For this review, take the finished solid that the model builds, in its own axes (mm). A direction names the side the tool comes from. Round coordinates to 2 decimals unless told otherwise and drop trailing zeros. Loops run counter-clockwise (first coordinate to the right, second up) from the corner with the lowest first, then second, coordinate; pieces in that order, holes last.
1) Mouldability with a two-part tool opening along X and no side actions: class faces 1 (the cylindrical face through (21.107, 38.24, 23.706)), 2 (the flat face through (24.237, 75, 21)), 3 (the flat face through (-20.213, 75, 20)) as pulls with the +X half, pulls with the -X half, needs draft (parallel to the pull), parting line crosses it, or undercut.
2) Take a section at A-A (x = -16.5). State the section outline as (y, z) points, then the cut area to 3 significant figures.
3) Take a section at B-B (y = 63.5). State the section outline as (x, z) points.
4) Take a section at D-D (z = 21.75). Give the number of separate pieces and of enclosed holes in the cut face, then the cut area to 3 significant figures.
5) Wall thickness on L1, parallel to Z at x = -18.5, y = 55.5; L2, parallel to X at y = 126, z = 17.75; L3, parallel to Z at x = -24, y = 12.5: over which ranges is each line inside the solid? List them lowest first.
6) Take a section at C-C (y = 24). State the section outline as (x, z) points, then the cut area to 3 significant figures.
7) Tool access review of faces 4 (the cylindrical face through (21.11, 85.8, 21.22)), 5 (the flat face through (-1, 75, 26.884)): name each direction out of +Z, -Z, +X, -X, +Y, -Y from which nothing blocks a thin tool from reaching the whole face with its end or side.
Autodesk Inventor part; units mm, degrees
ref_plane "YZ Plane" through (0, 0, 0) normal (1, 0, 0) x (0, 1, 0)
ref_plane "XZ Plane" through (0, 0, 0) normal (0, 1, 0) x (-1, 0, 0)
ref_plane "XY Plane" through (0, 0, 0) normal (0, 0, 1) x (1, 0, 0)
sketch "Sketch1" plane through (0, 0, 0) normal (0, 1, 0) x (-1, 0, 0)
  line L0 (-24.2371, 7.8342) -> (26.5629, 7.8342)
  line L1 (26.5629, 7.8342) -> (26.5629, 33.2342)
  line L2 (26.5629, 33.2342) -> (-24.2371, 33.2342)
  line L3 (-24.2371, 33.2342) -> (-24.2371, 7.8342)
  line L4 (-17.8871, 14.1842) -> (20.2129, 14.1842)
  line L5 (20.2129, 14.1842) -> (20.2129, 26.8842)
  line L6 (20.2129, 26.8842) -> (-17.8871, 26.8842)
  line L7 (-17.8871, 26.8842) -> (-17.8871, 14.1842)
  point P0 (0, 0)
  dimension "d0" = 50.8
  dimension "d1" = 25.4
  dimension "d2" = 6.35
extrude "Extrusion1" add sketch "Sketch1" along normal blind 152.4
sketch "Sketch2" plane through (24.2371, 0, 33.2342) normal (1, 0, 0) x (0, 0, -1)
  line L0 (19.05, 0) -> (6.35, 0)
  line L1 (12.7, 0) -> (12.7, 152.4) construction
  line L2 (6.35, 152.4) -> (19.05, 152.4)
  circle A0 centre (12.7, 12.7) radius 3.175
  circle A1 centre (12.7, 38.1) radius 3.175
  circle A2 centre (12.7, 63.5) radius 3.175
  circle A3 centre (12.7, 88.9) radius 3.175
  circle A4 centre (12.7, 114.3) radius 3.175
  circle A5 centre (12.7, 139.7) radius 3.175
  point P0 (33.2342, 0)
  dimension "d5" = 6.35
  dimension "d6" = 12.7
  dimension "d9" = 25.4
extrude "Extrusion2" cut sketch "Sketch2" against normal through all
properties part number "Front Frame"
Response:
1. face 1: needs draft
1. face 2: pulls with the +X half
1. face 3: undercut
2. outline: (0, 7.83) - (152.4, 7.83) - (152.4, 14.18) - (0, 14.18) - close; (0, 26.88) - (152.4, 26.88) - (152.4, 33.23) - (0, 33.23) - close
2. area: 1,940 mm2
3. outline: (-26.56, 7.83) - (24.24, 7.83) - (24.24, 17.36) - (17.89, 17.36) - (17.89, 14.18) - (-20.21, 14.18) - (-20.21, 17.36) - (-26.56, 17.36) - close; (-26.56, 23.71) - (-20.21, 23.71) - (-20.21, 26.88) - (17.89, 26.88) - (17.89, 23.71) - (24.24, 23.71) - (24.24, 33.23) - (-26.56, 33.23) - close
4. separate pieces: 14
4. enclosed holes: 0
4. area: 1,490 mm2
5. L1: z = 7.83 to 14.18, 26.88 to 33.23
5. L2: x = -26.56 to -20.21, 17.89 to 24.24
5. L3: z = 7.83 to 17.37, 23.7 to 33.23
6. outline: (-26.56, 7.83) - (24.24, 7.83) - (24.24, 33.23) - (-26.56, 33.23) - close; hole (-20.21, 14.18) - (17.89, 14.18) - (17.89, 26.88) - (-20.21, 26.88) - close
6. area: 806 mm2
7. face 4: +X, -X
7. face 5: +Y, -Y
